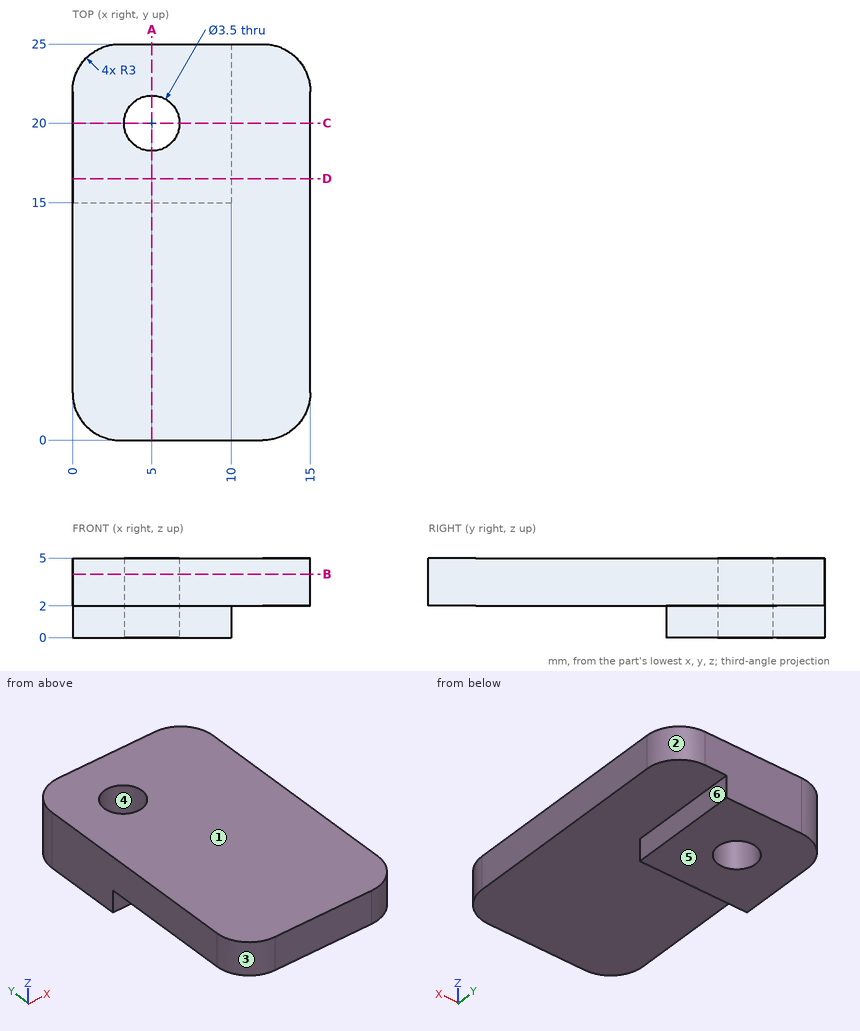
The drawing under review shows one solid part. Ordinate dimensions are in mm from its lowest x, y, z. A direction names the side the tool comes from. Round coordinates to 2 decimals unless told otherwise and drop trailing zeros. Loops run counter-clockwise (first coordinate to the right, second up) from the corner with the lowest first, then second, coordinate; pieces in that order, holes last. Notation, with made-up numbers: (69, -2.75) - (105, -2.75) arc R30 cw to (105, 34.25) - close; hole circle Ø3 at (60, 13.5). An arc over 180 degrees is marked (long way). Use a Markdown table: item, result. Add a question column.
Q1. Add section D-D (y = 16.5). State the section outline as (x, z) points, plus the area to 3 significant figures.
Q2. Add section C-C (y = 20). State the section outline as (x, z) points.
Q3. Add section B-B (z = 4). State the section outline as (x, y) points, plus the area to 3 significant figures.
Q4. Add section A-A (x = 5). State the section outline as (y, z) points, plus the area to 3 significant figures.
Q5. Insertion check: pin 1 Ø1 at (x, z) = (5, 1) entering from -Y; pin 2 Ø1 at (x, y) = (7, 12.5) entering from -Z; pin 3 Ø2 at (x, y) = (7, 18.5) entering from -Z; pin 4 Ø1 at (y, z) = (21.5, 0.5) entering from +X. Each pin has a flat end and moves straight along its axis. Give the tip position at first contact, or say it passes through.
Q6. Machinability: for the marked faces 5 and 6, which of the approach directions +Z, -Z, +X, -X, +Y, -Y give a long, thin tool a straight path to every point of the face, cutting with its end or side? Answer none if there is none.
Q7. The part is to be moulded in two halves that separate along Y. For the marked faces 1, 2, 3 and 4, say which applies: pulls with the +Y half, pulls with the -Y half, needs draft (parallel to the pull), parting line crosses it, or undercut.
Q8. For probe 1 along Y at (x, z) = (5, 3.45); probe 2 along Y at (x, z) = (9.75, 0.7); probe 3 along Z at (x, y) = (11, 6), list the stretches that pass through material, from the lowest coordinate up.
Worked answers:
| question | item | result |
|---|---|---|
| 1 | outline | (0, 0) - (10, 0) - (10, 2) - (15, 2) - (15, 5) - (0, 5) - close |
| 1 | area | 65.0 mm² |
| 2 | outline | (0, 0) - (3.25, 0) - (3.25, 5) - (0, 5) - close; (6.75, 0) - (10, 0) - (10, 2) - (15, 2) - (15, 5) - (6.75, 5) - close |
| 3 | outline | (0, 3) arc R3 ccw to (3, 0) - (12, 0) arc R3 ccw to (15, 3) - (15, 22) arc R3 ccw to (12, 25) - (3, 25) arc R3 ccw to (0, 22) - close; hole circle Ø3.5 at (5, 20) |
| 3 | area | 358 mm² |
| 4 | outline | (0, 2) - (15, 2) - (15, 0) - (18.25, 0) - (18.25, 5) - (0, 5) - close; (21.75, 0) - (25, 0) - (25, 5) - (21.75, 5) - close |
| 4 | area | 77.5 mm² |
| 5 | pin 1 | y = 15 |
| 5 | pin 2 | z = 2 |
| 5 | pin 3 | z = 0 |
| 5 | pin 4 | x = 10 |
| 6 | face 5 | -Z, +X, -X, +Y, -Y |
| 6 | face 6 | -Z, +X, +Y, -Y |
| 7 | face 1 | needs draft |
| 7 | face 2 | pulls with the +Y half |
| 7 | face 3 | pulls with the -Y half |
| 7 | face 4 | undercut |
| 8 | probe 1 | 0 to 18.25, 21.75 to 25 |
| 8 | probe 2 | 15 to 25 |
| 8 | probe 3 | 2 to 5 |
